Could you check a few things on this model? Use its own coordinates, in mm. Give positions to 0.01 mm unless a question says otherwise; leave off trailing zeros. Order: outer loops, then holes, each group sorted by start corner. A loop starts at its lowest first (then second) coordinate and runs counter-clockwise, first axis right, second up. Notation, with made-up numbers: M 0,86 L 41,86 A17 ccw 41,114 Z; hole C 47.5,-1.75 d10. An arc over 180 degrees is marked long. Return JSON: item names as keys, results as strings. Group by question number.
```python
from build123d import *

# Parameters (mm, degrees)
SKETCH1_W           = 170
SKETCH1_H           = 65
SKETCH1_R           = 1.6
BOSS_EXTRUDE1_DEPTH = 5


with BuildPart() as part:
    # Sketch1 → Boss-Extrude1 (new body)
    with BuildSketch(Plane(origin=(0, 0, 0), x_dir=(1, 0, 0), z_dir=(0, 1, 0))):
        Rectangle(SKETCH1_W, SKETCH1_H)
        with Locations((-82.5, 17.5)):
            Circle(SKETCH1_R, mode=Mode.SUBTRACT)
        with Locations((-82.5, -2.5)):
            Circle(SKETCH1_R, mode=Mode.SUBTRACT)
        with Locations((-82.5, -22.5)):
            Circle(SKETCH1_R, mode=Mode.SUBTRACT)
        with Locations((82.5, -22.5)):
            Circle(SKETCH1_R, mode=Mode.SUBTRACT)
        with Locations((82.5, -2.5)):
            Circle(SKETCH1_R, mode=Mode.SUBTRACT)
        with Locations((82.5, 17.5)):
            Circle(SKETCH1_R, mode=Mode.SUBTRACT)
    extrude(amount=BOSS_EXTRUDE1_DEPTH)


solid = part.part
```
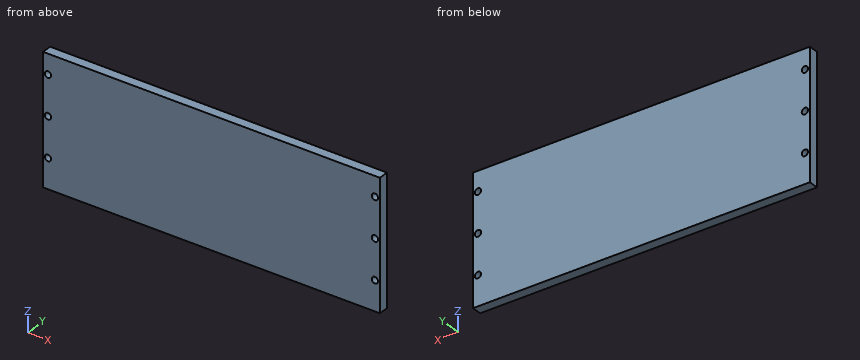
1. Imagine slicing it at B-B, the plane x = 82.5. Please give me the cut outline in (y, z).
2. Imagine slicing it at A-A, the plane z = 22.5. Please give me the cut outline in (x, y), plus the area to 3 significant figures.
3. I need wall thicknesses on L1, parallel to Z at x = 82.5, y = 3.55; L2, parallel to X at y = 2.1, z = 22.5; L3, parallel to X at y = 3.3, z = 22. Which ranges of each line are inside material? Lowest first, please. Write a range as from..to.
Values:
{
 "1": {"outline": "M 0,-32.5 L 5,-32.5 L 5,-19.1 L 0,-19.1 Z; M 0,-15.9 L 5,-15.9 L 5,0.9 L 0,0.9 Z; M 0,4.1 L 5,4.1 L 5,20.9 L 0,20.9 Z; M 0,24.1 L 5,24.1 L 5,32.5 L 0,32.5 Z"},
 "2": {"outline": "M -85,0 L -84.1,0 L -84.1,5 L -85,5 Z; M -80.9,0 L 80.9,0 L 80.9,5 L -80.9,5 Z; M 84.1,0 L 85,0 L 85,5 L 84.1,5 Z", "area": "818 mm²"},
 "3": {"L1": "z = -32.5..-19.1, -15.9..0.9, 4.1..20.9, 24.1..32.5", "L2": "x = -85..-84.1, -80.9..80.9, 84.1..85", "L3": "x = -85..-84.02, -80.98..80.98, 84.02..85"}
}
